Check sheet for the drawn part. Datum: minimum x, y, z corner. Units: mm. A direction names the side the tool comes from. Coordinates: 2 decimals unless noted, no trailing zeros. Order: outer loops, then holes, each group sorted by start corner. A loop starts at its lowest first (then second) coordinate and runs counter-clockwise, first axis right, second up. Notation, with made-up numbers: M 74.5,79 L 78.5,79 A19 cw 78.5,95 Z; hole C 5.5,-33.75 d4. An arc over 180 degrees is marked long. Return JSON: item names as keys, results as strings. Group by question number.
Q1. Section check B-B, the plane z = 62. Enter the section's corners in (x, y).
Q2. Access from +Z, -Z, +X, -X, +Y, -Y to the whole of each face (thin tool, end or side, straight path). Record for the marked faces 1, 2 and 3.
Q3. Section check A-A, the plane x = 70. Enter the section's corners in (y, z) (1 decimal).
Q4. Section check C-C, the plane y = 54. Enter the section's corners in (x, z) (1 decimal).
Q5. Go/stop test with flat-tipped pins: pin 1 Ø2 at (y, z) = (69.5, 84.5) entering from +X; pin 2 Ø12 at (x, y) = (89.5, 45) entering from +Z; pin 3 Ø6 at (x, z) = (26.5, 102) entering from +Y. Record where each tip stops, or that it passes through.
Q6. Section check D-D, the plane z = 41. Enter the section's corners in (x, y) (1 decimal).
Q7. Thickness scan on probe 1 along X at (y, z) = (29, 54); probe 2 along Y at (x, z) = (151, 27.5); probe 3 along Z at (x, y) = (65, 27.5) (1 decimal). Record the ranges inside material, lowest first.
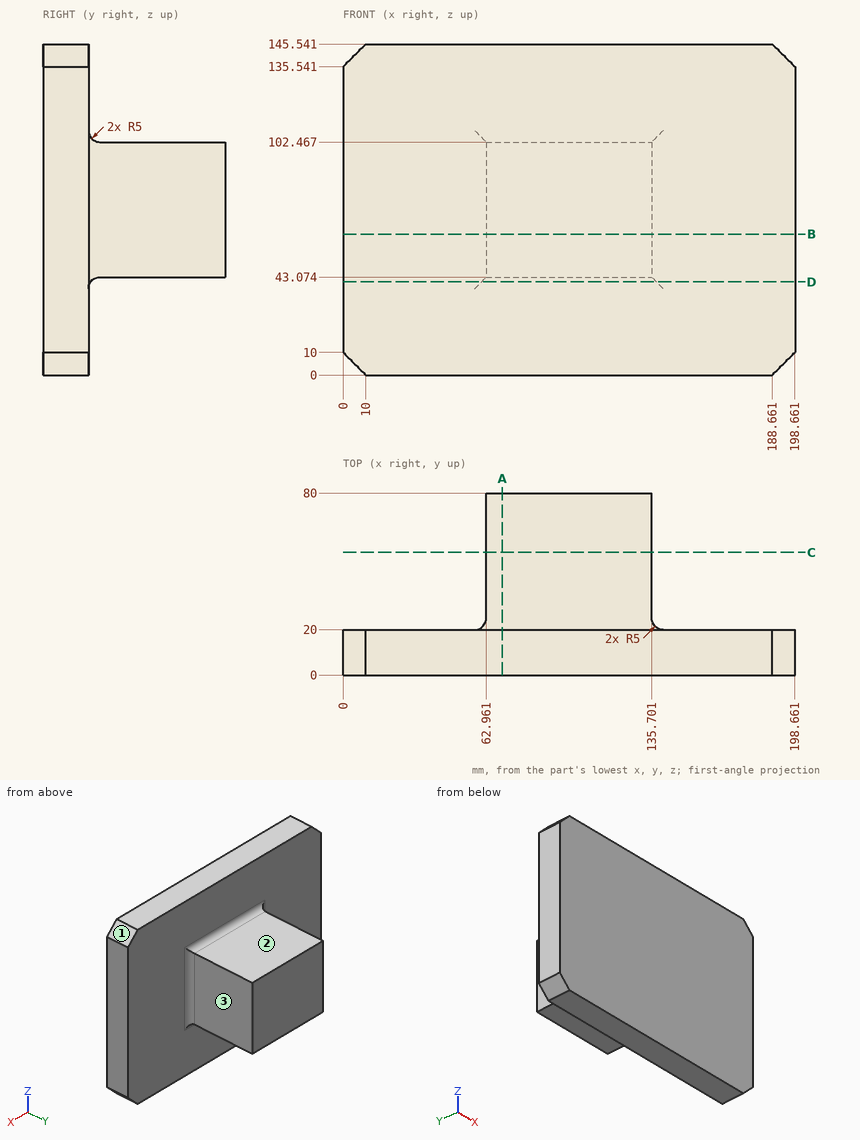
Numbers:
{
 "1": {"outline": "M 0,0 L 198.66,0 L 198.66,20 L 140.7,20 A5 cw 135.7,25 L 135.7,80 L 62.96,80 L 62.96,25 A5 cw 57.96,20 L 0,20 Z"},
 "2": {"face 1": "+Z, +X, +Y, -Y", "face 2": "+Z, +X, -X, +Y", "face 3": "+Z, -Z, +X, +Y"},
 "3": {"outline": "M 0,0 L 20,0 L 20,38.1 A5 cw 25,43.1 L 80,43.1 L 80,102.5 L 25,102.5 A5 cw 20,107.5 L 20,145.5 L 0,145.5 Z"},
 "4": {"outline": "M 63,43.1 L 135.7,43.1 L 135.7,102.5 L 63,102.5 Z"},
 "5": {"pin 1": "stops at x = 135.7", "pin 2": "stops at z = 102.47", "pin 3": "stops at y = 20"},
 "6": {"outline": "M 0,0 L 198.7,0 L 198.7,20 L 140.7,20 A5 cw 137.8,20.9 L 60.9,20.9 A5 cw 58,20 L 0,20 Z"},
 "7": {"probe 1": "x = 62.96 to 135.7", "probe 2": "y = 0 to 20", "probe 3": "z = 43.1 to 102.5"}
}
